Part model, mm, in its own coordinate system. Face numbers are marked on the shaded views. A direction names the side the tool comes from. Round coordinates to 2 decimals unless told otherwise and drop trailing zeros. Order: outer loops, then holes, each group sorted by start corner. A loop starts at its lowest first (then second) coordinate and runs counter-clockwise, first axis right, second up. Notation, with made-up numbers: (-27, 35.25) -> (-19, 35.25) arc R24 ccw to (-19, 61.25) -> close; hole circle Ø3 at (24, 86.25). An arc over 180 degrees is marked (long way). Use CSV: the item, a comma, the result in double quotes.
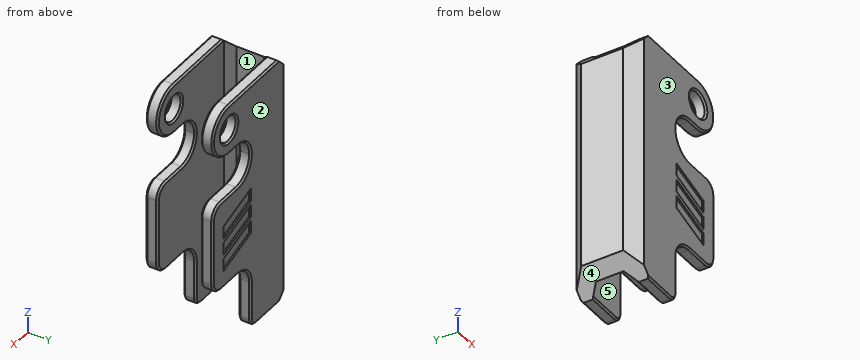
```python
from build123d import *

# Parameters (mm, degrees)
SKETCH_1_W          = 29
SKETCH_1_H          = 60
EXTRUDE_1_DEPTH     = 16
SKETCH_2_W          = 26.2
SKETCH_2_H          = 10.2
CUT_EXTRUDE_1_DEPTH = 69.534662763
SKETCH_3_R          = 3
CUT_EXTRUDE_2_DEPTH = 69.534662763
CUT_EXTRUDE_3_DEPTH = 69.534662763
CUT_EXTRUDE_4_DEPTH = 69.534662763
CUT_EXTRUDE_5_DEPTH = 69.534662763
FILLET_1_R          = 3
CHAMFER_1_SIZE      = 5
CHAMFER_3_SIZE      = 3
CHAMFER_4_SIZE      = 1.8
FILLET_2_R          = 2
CHAMFER_2_SIZE      = 0.4
CUT_EXTRUDE_6_DEPTH = 0.4


with BuildPart() as part:
    # 草图1 → 凸台-拉伸1 (new body)
    with BuildSketch(Plane(origin=(0, 0, 0), x_dir=(1, 0, 0), z_dir=(0, 1, 0))):
        with Locations((14.5, 30)):
            Rectangle(SKETCH_1_W, SKETCH_1_H)
    extrude(amount=EXTRUDE_1_DEPTH)

    # 草图2 → 切除-拉伸1 (cut, through all)
    with BuildSketch(Plane(origin=(0, 0, -60), x_dir=(-1, 0, 0), z_dir=(0, 0, -1))):
        with Locations((-15.9, 8)):
            Rectangle(SKETCH_2_W, SKETCH_2_H)
    extrude(amount=-CUT_EXTRUDE_1_DEPTH, mode=Mode.SUBTRACT)

    # 草图3 → 切除-拉伸2 (cut, through all)
    with BuildSketch(Plane(origin=(0, 0, 0), x_dir=(-1, 0, 0), z_dir=(0, -1, 0))):
        with Locations(Location((-23, 6, 0), (0, 0, 90))):
            Circle(SKETCH_3_R)
    extrude(amount=-CUT_EXTRUDE_2_DEPTH, mode=Mode.SUBTRACT)

    # 草图4 → 切除-拉伸3 (cut, through all)
    with BuildSketch(Plane(origin=(0, 16, 0), x_dir=(1, 0, 0), z_dir=(0, 1, 0))):
        with BuildLine():
            Line((23, 0), (24.972936344, -1.282691022))
            Line((24.972936344, -1.282691022), (32.744307438, -1.586182692))
            Line((32.744307438, -1.586182692), (32.104431406, 9.686424342))
            Line((32.104431406, 9.686424342), (29.958145659, 12))
            Line((29.958145659, 12), (23, 12))
            ThreePointArc((23, 12), (29, 6), (23, 0))
        make_face()
    extrude(amount=-CUT_EXTRUDE_3_DEPTH, mode=Mode.SUBTRACT)

    # 草图5 → 切除-拉伸4 (cut, through all)
    with BuildSketch(Plane(origin=(0, 16, 0), x_dir=(1, 0, 0), z_dir=(0, 1, 0))):
        with BuildLine():
            Line((29, 12), (19.99, 12))
            ThreePointArc((19.99, 12), (16.461537162, 13.461537162), (15, 16.99))
            Line((15, 16.99), (15, 17.21))
            ThreePointArc((15, 17.21), (16.461537162, 20.738462838), (19.99, 22.2))
            Line((19.99, 22.2), (29, 22.2))
            Line((29, 22.2), (29, 12))
        make_face()
    extrude(amount=-CUT_EXTRUDE_4_DEPTH, mode=Mode.SUBTRACT)

    # 草图6 → 切除-拉伸5 (cut, through all)
    with BuildSketch(Plane(origin=(0, 16, 0), x_dir=(1, 0, 0), z_dir=(0, 1, 0))):
        with BuildLine():
            Line((29, 60), (15, 60))
            Line((15, 60), (15, 48.8))
            ThreePointArc((15, 48.8), (16.464466094, 45.264466094), (20, 43.8))
            Line((20, 43.8), (29, 43.8))
            Line((29, 43.8), (29, 60))
        make_face()
    extrude(amount=-CUT_EXTRUDE_5_DEPTH, mode=Mode.SUBTRACT)

    # 圆角1
    fillet_1_edges = [part.edges().sort_by_distance(p)[0] for p in [
        (29, 14.55, -43.8),
        (29, 1.45, -43.8),
        (29, 14.55, -22.2),
        (29, 1.45, -22.2),
    ]]
    fillet(fillet_1_edges, radius=FILLET_1_R)

    # 倒角1
    # the kernel refuses this chamfer: 5 mm, written as the material it takes off along each edge
    with BuildSketch(Plane(origin=(0, -12.85841494, -60), x_dir=(0.9996219169112968, 0, -0.027495876610586317), z_dir=(0, 1, 0)), Plane(origin=(0, -12.85841494, 0), x_dir=(-0.027495876610586372, 0, -0.9996219169112968), z_dir=(0, 1, 0))) as chamfer_1_piece_1:
        Polygon((CHAMFER_1_SIZE * 0.999621916911, -CHAMFER_1_SIZE * 0.0274958766106), (-CHAMFER_1_SIZE * 0.0274958766106, -CHAMFER_1_SIZE * 0.999621916911), (0, 0), align=None)
    extrude(amount=41.71682988, mode=Mode.SUBTRACT)

    # 倒角3
    chamfer_3_edges = [part.edges().sort_by_distance(p)[0] for p in [
        (0, 0, -30),
        (0, 16, -30),
    ]]
    chamfer(chamfer_3_edges, length=CHAMFER_3_SIZE)

    # 倒角4
    chamfer_4_edges = [part.edges().sort_by_distance(p)[0] for p in [
        (2.8, 13.1, -30),
        (2.8, 2.9, -30),
    ]]
    chamfer(chamfer_4_edges, length=CHAMFER_4_SIZE)

    # 圆角2
    fillet_2_edges = [part.edges().sort_by_distance(p)[0] for p in [
        (15, 14.55, -60),
        (15, 1.45, -60),
    ]]
    fillet(fillet_2_edges, radius=FILLET_2_R)

    # 倒角2
    chamfer_2_edges = [part.edges().sort_by_distance(p)[0] for p in [
        (23, 0, -3),
        (29, 0, -6),
        (21.495, 0, -12),
        (16.461537162, 0, -13.461537162),
        (15, 0, -17.1),
        (16.461537162, 0, -20.738462838),
        (22.995, 0, -22.2),
        (28.121320344, 0, -23.078679656),
        (29, 0, -33),
        (28.121320344, 0, -42.921320344),
        (23, 0, -43.8),
        (16.464466094, 0, -45.264466094),
        (15, 0, -53.4),
        (9, 0, -60),
        (14, 0, 0),
        (29, 13.1, -6),
        (21.495, 13.1, -12),
        (16.461537162, 13.1, -13.461537162),
        (15, 13.1, -17.1),
        (16.461537162, 13.1, -20.738462838),
        (22.995, 13.1, -22.2),
        (28.121320344, 13.1, -23.078679656),
        (29, 13.1, -33),
        (28.121320344, 13.1, -42.921320344),
        (23, 13.1, -43.8),
        (16.464466094, 13.1, -45.264466094),
        (15, 13.1, -53.4),
        (9, 13.1, -60),
        (14, 13.1, 0),
        (23, 13.1, -3),
        (9, 2.9, -60),
        (15, 2.9, -53.4),
        (16.464466094, 2.9, -45.264466094),
        (23, 2.9, -43.8),
        (28.121320344, 2.9, -42.921320344),
        (29, 2.9, -33),
        (28.121320344, 2.9, -23.078679656),
        (22.995, 2.9, -22.2),
        (16.461537162, 2.9, -20.738462838),
        (15, 2.9, -17.1),
        (16.461537162, 2.9, -13.461537162),
        (21.495, 2.9, -12),
        (29, 2.9, -6),
        (14, 2.9, 0),
        (23, 2.9, -3),
        (9, 16, -60),
        (15, 16, -53.4),
        (16.464466094, 16, -45.264466094),
        (23, 16, -43.8),
        (28.121320344, 16, -42.921320344),
        (29, 16, -33),
        (28.121320344, 16, -23.078679656),
        (22.995, 16, -22.2),
        (16.461537162, 16, -20.738462838),
        (15, 16, -17.1),
        (16.461537162, 16, -13.461537162),
        (21.495, 16, -12),
        (29, 16, -6),
        (14, 16, 0),
        (23, 16, -3),
        (14.414213562, 0, -59.414213562),
        (14.414213562, 13.1, -59.414213562),
        (14.414213562, 2.9, -59.414213562),
        (14.414213562, 16, -59.414213562),
    ]]
    chamfer(chamfer_2_edges, length=CHAMFER_2_SIZE)

    # 草图7 → 切除-拉伸6 (cut)
    with BuildSketch(Plane(origin=(0, 16, 0), x_dir=(1, 0, 0), z_dir=(0, 1, 0))):
        Polygon((25, 28.7), (15, 25.498437881), (15, 28.498437881), (25, 31.7), align=None)
        Polygon((25, 32.7), (15, 29.498437881), (15, 32.498437881), (25, 35.7), align=None)
        Polygon((25, 36.7), (15, 33.498437881), (15, 36.498437881), (25, 39.7), align=None)
    cut_extrude_6 = extrude(amount=-CUT_EXTRUDE_6_DEPTH, mode=Mode.SUBTRACT)

    # 镜向1: 切除-拉伸6 across plane
    add(cut_extrude_6.mirror(Plane.ZX.offset(8)), mode=Mode.SUBTRACT)


solid = part.part
```
(1) Pull direction Y, two halves, no side cores. Call the marked faces 3, 4 and 5: released by +Y, released by -Y, zero draft, split by the parting line, or undercut.
Reply:
face 3,"released by -Y"
face 4,"zero draft"
face 5,"undercut"
(2) Which spindle directions (+Z, -Z, +X, -X, +Y, -Y) get a long thin tool onto all of the face, cutting with end or side? Do the marked faces 1 and 2. Say none if no direction does.
Reply:
face 1,"+Z, -Z, +X"
face 2,"+Z, -Z, +X, -X, +Y"
(3) Cut at B-B, the plane y = 1.75. Give the cut face in (x, z).
Reply:
outline,"(1.25, -56.25) -> (5, -60) -> (13, -60) arc R2 ccw to (15, -58) -> (15, -48.8) arc R5 cw to (20, -43.8) -> (26, -43.8) arc R3 ccw to (29, -40.8) -> (29, -25.2) arc R3 ccw to (26, -22.2) -> (19.99, -22.2) arc R4.99 cw to (15, -17.21) -> (15, -16.99) arc R4.99 cw to (19.99, -12) -> (23, -12) arc R6 ccw to (23, 0) -> (5, 0) -> (1.25, -3.75) -> close; hole circle Ø6 at (23, -6)"
(4) Cut at A-A, the plane z = -6. State how many separate pieces and enclosed holes the cut face has, then the cut area to 3 significant figures.
Reply:
separate pieces,"3"
enclosed holes,"0"
area,"155 mm2"
(5) Probe probe 1 along Z at (x, y) = (22.75, 2.25); probe 2 along Y at (x, z) = (9.75, -51); probe 3 along Z at (x, y) = (24.25, 14.25). List the from-to ranges inside material, lowest first. Write a range as [from, to].
Reply:
probe 1,"[-43.8, -22.2], [-12, -8.99], [-3.01, 0]"
probe 2,"[0, 2.9], [13.1, 16]"
probe 3,"[-43.8, -22.2], [-11.87, -8.73], [-3.27, -0.13]"
(6) Drop flat-ended pins along their axis: P1, Ø1.1, axis at y = 1, z = -51.5, coming from the +X side; P2, Ø2.5, axis at x = 22.5, y = 14.5, coming from the -Z side; P3, Ø3, axis at y = 10.5, z = -24, coming from the +X side; P4, Ø2, axis at x = 24, y = 4.5, coming from the -Z side (1 decimal). Give the stop position or say it passes through.
Reply:
P1,"x = 15"
P2,"z = -43.8"
P3,"x = 3.5"
P4,"through"
(7) Cut at D-D, the plane y = 6.75. Give the cut face in (x, z).
Reply:
outline,"(0, -55) -> (2.8, -57.8) -> (2.8, -2.2) -> (0, -5) -> close"
